Work out the finished part from the listing and answer in its coordinate system (mm). Give positions to 0.01 mm unless a question says otherwise; leave off trailing zeros. Loops run counter-clockwise (first coordinate to the right, second up) from the corner with the lowest first, then second, coordinate; pieces in that order, holes last.
from build123d import *

# Parameters (mm, degrees)
F0_W     = 279.4
F0_H     = 381
F1_DEPTH = 3.556
F2_W     = 167.639992
F2_H     = 269.239992
F3_DEPTH = 56.388
F4_R     = 172.737905
F5_DEPTH = 141.843393


with BuildPart() as f1:
    # F0 (on Right) → F1 (new body)
    with BuildSketch(Plane.YZ):
        Rectangle(F0_W, F0_H)
    extrude(amount=-F1_DEPTH)

    # F2 (on face) → F3 (cut)
    with BuildSketch(Plane(origin=(-3.556, 0, 0), x_dir=(0, -1, 0), z_dir=(-1, 0, 0))):
        Rectangle(F2_W, F2_H)
    extrude(amount=-F3_DEPTH, mode=Mode.SUBTRACT)

    # F4 (on Front) → F5 (join)
    with BuildSketch(Plane.XZ):
        Circle(F4_R)
    extrude(amount=F5_DEPTH)


solid = f1.part
Item 1: Find section C-C, the plane y = -80.5. Write down the section's boundary in (x, z).
Item 2: Consider line 1 (Y direction, x = -21, z = 166.5); line 2 (X direction, y = -90, z = 174); line 3 (Z direction, x = 82, y = -22). Determine where each line is inside the solid, lowest interval first.
Item 3: Find section B-B, the plane z = 0. Write down the section's boundary in (x, y), plus the area to 3 significant figures.
Item 4: Flat-ended cylindrical pins translate along their axes: pin 1 Ø4 at (x, z) = (-1.5, 180.5) entering from -Y; pin 2 Ø12 at (y, z) = (24, 150) entering from -X; pin 3 Ø4 at (x, z) = (-100, -38) entering from +Y. Find the tip coordinate at first contact, or state that the pin passes through.
Item 5: Find section D-D, the plane z = 161. Write down the section's boundary in (x, y).
Item 6: Find section A-A, the plane y = 33.5. Write down the section's boundary in (x, z), plus the area to 3 significant figures.
Ans:
1. outline: (-3.56, -190.5) - (0, -190.5) - (0, -172.74) arc R172.74 ccw to (0, 172.74) - (0, 190.5) - (-3.56, 190.5) - (-3.56, 172.7) arc R172.74 ccw to (-3.56, -172.7) - close
2. line 1: y = -141.84 to 0
2. line 2: x = -3.56 to 0
2. line 3: z = -152.03 to 152.03
3. outline: (-172.74, -141.84) - (172.74, -141.84) - (172.74, 0) - (-172.74, 0) - close; (-3.56, 83.82) - (0, 83.82) - (0, 139.7) - (-3.56, 139.7) - close
3. area: 49,200 mm2
4. pin 1: stops at y = -139.7
4. pin 2: stops at x = -3.56
4. pin 3: stops at y = 0
5. outline: (-62.59, -141.84) - (62.59, -141.84) - (62.59, 0) - (0, 0) - (0, 139.7) - (-3.56, 139.7) - (-3.56, 0) - (-62.59, 0) - close
6. outline: (-3.56, -190.5) - (0, -190.5) - (0, -134.62) - (-3.56, -134.62) - close; (-3.56, 134.62) - (0, 134.62) - (0, 190.5) - (-3.56, 190.5) - close
6. area: 397 mm2
